For this review, take the finished solid that the model builds, in its own axes (mm). Face numbers are marked on the shaded views. Give positions to 0.01 mm unless a question says otherwise; leave off trailing zeros. Loops run counter-clockwise (first coordinate to the right, second up) from the corner with the lowest first, then second, coordinate; pieces in that order, holes last.
```python
from build123d import *

# Parameters (mm, degrees)
SKETCH1_W           = 190
SKETCH1_H           = 65
SKETCH1_R           = 2.1
BOSS_EXTRUDE1_DEPTH = 2.2
SKETCH3_W           = 5.822409575
SKETCH3_H           = 15.664234042
SKETCH3_W_2         = 5.822409574
SKETCH3_H_2         = 39.034260638
BOSS_EXTRUDE3_DEPTH = 1.4
FILLET1_R           = 10


with BuildPart() as part:
    # Sketch1 → Boss-Extrude1 (new body)
    with BuildSketch(Plane(origin=(0, 0, 0), x_dir=(1, 0, 0), z_dir=(0, 1, 0))):
        Rectangle(SKETCH1_W, SKETCH1_H)
        with Locations(Location((-88, 7.623179707, 0), (0, 0, 270))):
            Circle(SKETCH1_R, mode=Mode.SUBTRACT)
        with Locations(Location((-88, -24.376820293, 0), (0, 0, 270))):
            Circle(SKETCH1_R, mode=Mode.SUBTRACT)
        with Locations(Location((88, -24.376820293, 0), (0, 0, 90))):
            Circle(SKETCH1_R, mode=Mode.SUBTRACT)
        with Locations(Location((88, 7.623179707, 0), (0, 0, 90))):
            Circle(SKETCH1_R, mode=Mode.SUBTRACT)
    extrude(amount=BOSS_EXTRUDE1_DEPTH)

    # Sketch3 → Boss-Extrude3 (add)
    # profile 1 of 5: a face of its own
    with BuildSketch(Plane(origin=(0, 2.2, 0), x_dir=(1, 0, 0), z_dir=(0, 1, 0))):
        Polygon((-77.439519604, 20.61757665), (-77.439519604, 27.58839048), (-64.531455774, 27.58839048), (-64.531455774, -26.857455265), (-73.42010471, -26.857455265), (-73.42010471, 19.882597927), (-75.234583434, 19.882597927), align=None)
    # profile 2 of 5: a face of its own
    with BuildSketch(Plane(origin=(0, 2.2, 0), x_dir=(1, 0, 0), z_dir=(0, 1, 0))):
        with BuildLine():
            Line((-34.778598327, 8.984241544), (-34.778598327, 19.882597927))
            Line((-34.778598327, 19.882597927), (-40.601007902, 19.882597927))
            Line((-40.601007902, 19.882597927), (-40.601007902, 4.218363884))
            Line((-40.601007902, 4.218363884), (-31.367837689, 4.218363884))
            add(Edge.make_bspline(
                [(-31.367837689, 4.218363884), (-30.937734177, 4.205882557), (-30.126413548, 4.182338553), (-28.991073812, 3.931040784), (-28.02102206, 3.502870767), (-27.219902727, 2.897866579), (-26.601465528, 2.109735687), (-26.1809682, 1.150054083), (-25.910893392, 0.033711404), (-25.889664372, -0.767797312), (-25.878465349, -1.190620158)],
                knots=[0, 0, 0, 0, 1.167027584, 2.201408559, 3.136967793, 4.027212192, 4.901025933, 5.82711576, 6.853730371, 8, 8, 8, 8], degree=3))
            Line((-25.878465349, -1.190620158), (-25.878465349, -21.448471222))
            add(Edge.make_bspline(
                [(-25.878465349, -21.448471222), (-25.889664372, -21.871294068), (-25.910893392, -22.672802785), (-26.1809682, -23.789145463), (-26.601465528, -24.748827067), (-27.219902727, -25.53695796), (-28.02102206, -26.141962147), (-28.991073812, -26.570132165), (-30.126413548, -26.821429933), (-30.937734177, -26.844973937), (-31.367837689, -26.857455265)],
                knots=[0, 0, 0, 0, 1.146269629, 2.17288424, 3.098974067, 3.972787808, 4.863032207, 5.798591441, 6.832972416, 8, 8, 8, 8], degree=3))
            Line((-31.367837689, -26.857455265), (-44.746747264, -26.857455265))
            add(Edge.make_bspline(
                [(-44.746747264, -26.857455265), (-45.119703537, -26.844982711), (-45.825659581, -26.821373845), (-46.813372336, -26.566574969), (-47.656481489, -26.137409968), (-48.33959709, -25.520537859), (-48.870362201, -24.736796043), (-49.228799232, -23.781135063), (-49.463163603, -22.669394461), (-49.48049008, -21.870915209), (-49.489656838, -21.448471222)],
                knots=[0, 0, 0, 0, 1.084734094, 2.05325569, 2.94625814, 3.815111374, 4.706091482, 5.677498929, 6.771255973, 8, 8, 8, 8], degree=3))
            Line((-49.489656838, -21.448471222), (-49.489656838, 22.179406438))
            add(Edge.make_bspline(
                [(-49.489656838, 22.179406438), (-49.48049008, 22.601850424), (-49.463163603, 23.400329677), (-49.228799232, 24.512070279), (-48.870362201, 25.467731259), (-48.33959709, 26.251473075), (-47.656481489, 26.868345184), (-46.813372336, 27.297510184), (-45.825659581, 27.55230906), (-45.119703537, 27.575917926), (-44.746747264, 27.58839048)],
                knots=[0, 0, 0, 0, 1.228744027, 2.322501071, 3.293908518, 4.184888626, 5.05374186, 5.94674431, 6.915265906, 8, 8, 8, 8], degree=3))
            Line((-44.746747264, 27.58839048), (-31.367837689, 27.58839048))
            add(Edge.make_bspline(
                [(-31.367837689, 27.58839048), (-30.937734177, 27.575909152), (-30.126413548, 27.552365149), (-28.991073812, 27.30106738), (-28.02102206, 26.872897363), (-27.219902727, 26.267893175), (-26.601465528, 25.479762283), (-26.1809682, 24.520080679), (-25.910893392, 23.403738), (-25.889664372, 22.602229284), (-25.878465349, 22.179406438)],
                knots=[0, 0, 0, 0, 1.167027584, 2.201408559, 3.136967793, 4.027212192, 4.901025933, 5.82711576, 6.853730371, 8, 8, 8, 8], degree=3))
            Line((-25.878465349, 22.179406438), (-25.878465349, 8.984241544))
            Line((-25.878465349, 8.984241544), (-34.778598327, 8.984241544))
        make_face()
        with Locations((-37.689803115, -11.31954569)):
            Rectangle(SKETCH3_W, SKETCH3_H, mode=Mode.SUBTRACT)
    # profile 3 of 5: a face of its own
    with BuildSketch(Plane(origin=(0, 2.2, 0), x_dir=(1, 0, 0), z_dir=(0, 1, 0))):
        Polygon((-11.732421732, 20.61757665), (-11.732421732, 27.58839048), (1.175642098, 27.58839048), (1.175642098, -26.857455265), (-7.713006838, -26.857455265), (-7.713006838, 19.882597927), (-9.527485561, 19.882597927), align=None)
    # profile 4 of 5: a face of its own
    with BuildSketch(Plane(origin=(0, 2.2, 0), x_dir=(1, 0, 0), z_dir=(0, 1, 0))):
        Polygon((32.398456992, 27.220901118), (39.828632524, 27.58839048), (39.828632524, -26.857455265), (30.928499545, -26.857455265), (30.928499545, -14.397269094), (14.873808056, -14.397269094), (20.305760183, 27.58839048), (29.125504864, 27.58839048), (24.577824013, -6.691476541), (30.928499545, -6.691476541), (30.928499545, 26.853411757), align=None)
    # profile 5 of 5: a face of its own
    with BuildSketch(Plane(origin=(0, 2.2, 0), x_dir=(1, 0, 0), z_dir=(0, 1, 0))):
        with BuildLine():
            add(Edge.make_bspline(
                [(73.440128268, 27.58839048), (73.870231781, 27.575909152), (74.68155241, 27.552365149), (75.816892146, 27.30106738), (76.786943898, 26.872897363), (77.58806323, 26.267893175), (78.20650043, 25.479762283), (78.626997757, 24.520080679), (78.897072565, 23.403738), (78.918301585, 22.602229284), (78.929500609, 22.179406438)],
                knots=[0, 0, 0, 0, 1.167027584, 2.201408559, 3.136967793, 4.027212192, 4.901025933, 5.82711576, 6.853730371, 8, 8, 8, 8], degree=3))
            Line((78.929500609, 22.179406438), (78.929500609, -21.448471222))
            add(Edge.make_bspline(
                [(78.929500609, -21.448471222), (78.918301585, -21.871294068), (78.897072565, -22.672802785), (78.626997757, -23.789145463), (78.20650043, -24.748827067), (77.58806323, -25.53695796), (76.786943898, -26.141962147), (75.816892146, -26.570132165), (74.68155241, -26.821429933), (73.870231781, -26.844973937), (73.440128268, -26.857455265)],
                knots=[0, 0, 0, 0, 1.146269629, 2.17288424, 3.098974067, 3.972787808, 4.863032207, 5.798591441, 6.832972416, 8, 8, 8, 8], degree=3))
            Line((73.440128268, -26.857455265), (60.061218694, -26.857455265))
            add(Edge.make_bspline(
                [(60.061218694, -26.857455265), (59.688262421, -26.844982711), (58.982306376, -26.821373845), (57.994593622, -26.566574969), (57.151484468, -26.137409968), (56.468368867, -25.520537859), (55.937603756, -24.736796043), (55.579166725, -23.781135063), (55.344802355, -22.669394461), (55.327475878, -21.870915209), (55.318309119, -21.448471222)],
                knots=[0, 0, 0, 0, 1.084734094, 2.05325569, 2.94625814, 3.815111374, 4.706091482, 5.677498929, 6.771255973, 8, 8, 8, 8], degree=3))
            Line((55.318309119, -21.448471222), (55.318309119, 22.179406438))
            add(Edge.make_bspline(
                [(55.318309119, 22.179406438), (55.327475878, 22.601850424), (55.344802355, 23.400329677), (55.579166725, 24.512070279), (55.937603756, 25.467731259), (56.468368867, 26.251473075), (57.151484468, 26.868345184), (57.994593622, 27.297510184), (58.982306376, 27.55230906), (59.688262421, 27.575917926), (60.061218694, 27.58839048)],
                knots=[0, 0, 0, 0, 1.228744027, 2.322501071, 3.293908518, 4.184888626, 5.05374186, 5.94674431, 6.915265906, 8, 8, 8, 8], degree=3))
            Line((60.061218694, 27.58839048), (73.440128268, 27.58839048))
        make_face()
        with Locations((67.118162843, 0.365467608)):
            Rectangle(SKETCH3_W_2, SKETCH3_H_2, mode=Mode.SUBTRACT)
    extrude(amount=BOSS_EXTRUDE3_DEPTH)

    # Fillet1
    fillet1_edges = [part.edges().sort_by_distance(p)[0] for p in [
        (95, 1.1, 32.5),
        (-95, 1.1, 32.5),
        (-95, 1.1, -32.5),
        (95, 1.1, -32.5),
    ]]
    fillet(fillet1_edges, radius=FILLET1_R)


solid = part.part
```
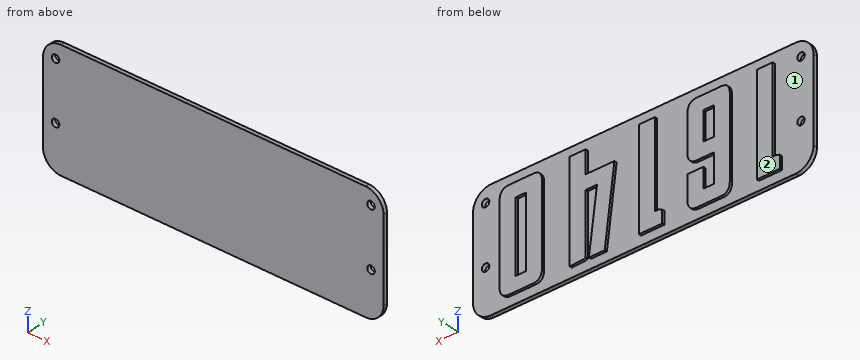
Q1. Consider section B-B on x = -88. Give the boundary of the cut face in (y, z).
Answers:
outline: (0, -32.04) - (2.2, -32.04) - (2.2, -9.72) - (0, -9.72) - close; (0, -5.52) - (2.2, -5.52) - (2.2, 22.28) - (0, 22.28) - close; (0, 26.48) - (2.2, 26.48) - (2.2, 32.04) - (0, 32.04) - close
Q2. Mouldability with a two-part tool opening along X and no side actions: class the marked faces 1 and 2 as +X half, -X half, draft (parallel to the pull), parting line (faces both ways), or undercut.
Answers:
face 1: undercut
face 2: draft
Q3. For probe 1 along X at (y, z) = (1.7, -9.5); probe 2 along Z at (x, y) = (88, 1.15); probe 3 along Y at (x, z) = (87.5, 11), list the stretches that pass through material, from the lowest coordinate up.
Answers:
probe 1: x = -95 to -88.94, -87.06 to 87.06, 88.94 to 95
probe 2: z = -32.04 to -9.72, -5.52 to 22.28, 26.48 to 32.04
probe 3: y = 0 to 2.2
Q4. Consider section A-A on y = 2.9. Count the separate pieces of the cut face and the enclosed holes in it, plus the area to 3 significant figures.
Answers:
separate pieces: 5
enclosed holes: 2
area: 4,010 mm2
Q5. Consider section D-D on x = 12.5. Give the boundary of the cut face in (y, z).
Answers:
outline: (0, -32.5) - (2.2, -32.5) - (2.2, 32.5) - (0, 32.5) - close
Q6. For pin 1 Ø0.7 at (x, y) = (22.5, 3) entering from -Z; pin 2 Ø0.7 at (y, z) = (3, 8) entering from -X; pin 3 Ø0.7 at (x, y) = (-38, 3) entering from +Z, all flat-tipped, find the tip position at first contact; note any pin that passes through.
Answers:
pin 1: stops at z = -27.59
pin 2: stops at x = -73.42
pin 3: stops at z = 26.86
